For this review, take the finished solid that the model builds, in its own axes (mm). Face numbers are marked on the shaded views. A direction names the side the tool comes from. Give positions to 0.01 mm unless a question says otherwise; leave off trailing zeros. Order: outer loops, then holes, each group sorted by start corner. A loop starts at its lowest first (then second) coordinate and runs counter-clockwise, first axis right, second up. Notation, with made-up numbers: M 21.5,64.5 L 47.5,64.5 A28 ccw 47.5,82.5 Z; hole C -23.5,36.5 d4. An arc over 180 degrees is marked long. Answer as CSV lines item,"result". Start each with the question number.
1. Clearance check with flat-ended pins moving along their axes: P1, Ø1.1, axis at y = 3, z = -6.5, coming from the -X side; P2, Ø3, axis at y = 4, z = -1.5, coming from the +X side; P3, Ø4, axis at y = 2.5, z = 2, coming from the -X side. State where each tip first meets the part, or that it passes through.
2. We need section B-B, the plane z = -1. State how many separate pieces and enclosed holes the cut face has, and give its area (3 significant figures).
3. Mouldability with a two-part tool opening along Z and no side actions: class the marked faces 4, 5 and 6 as pulls with the +Z half, pulls with the -Z half, needs draft (parallel to the pull), parting line crosses it, or undercut.
4. We need section A-A, the plane x = 28. Give the boundary of the cut face in (y, z), and give its area (3 significant figures).
5. For line 1 along Z through (x, y) = (-28.5, 3.25); line 2 along X through (y, z) = (2.25, 4); line 3 along X through (y, z) = (2.75, 1.75), list the stretches that pass through material, from the lowest coordinate up.
6. Machinability: for the marked faces 1, 2 and 3, which of the approach directions +Z, -Z, +X, -X, +Y, -Y give a long, thin tool a straight path to every point of the face, cutting with its end or side? Answer none if there is none.
from build123d import *

# Parameters (mm, degrees)
SKETCH1_W           = 70
SKETCH1_H           = 16
BOSS_EXTRUDE1_DEPTH = 7
CUT_EXTRUDE1_DEPTH  = 17
SKETCH3_R           = 2
BOSS_EXTRUDE2_DEPTH = 14
SKETCH4_W           = 39
SKETCH4_H           = 10
CUT_EXTRUDE2_DEPTH  = 2
FILLET1_R           = 1
FILLET2_R           = 3.5


with BuildPart() as part:
    # Sketch1 → Boss-Extrude1 (new body)
    with BuildSketch(Plane(origin=(0, 0, 0), x_dir=(1, 0, 0), z_dir=(0, 1, 0))):
        Rectangle(SKETCH1_W, SKETCH1_H)
    extrude(amount=BOSS_EXTRUDE1_DEPTH)

    # Sketch2 → Cut-Extrude1 (cut)
    with BuildSketch(Plane(origin=(0, 7, 0), x_dir=(1, 0, 0), z_dir=(0, 1, 0))):
        Polygon((-30, 7), (-35, 7), (-35, -7), (-30, -7), (-30, -5), (-23, -5), (-23, 5), (-30, 5), align=None)
        Polygon((30, -5), (30, -7), (35, -7), (35, 7), (30, 7), (30, 5), (23, 5), (23, -5), align=None)
    extrude(amount=-CUT_EXTRUDE1_DEPTH, mode=Mode.SUBTRACT)

    # Sketch3 → Boss-Extrude2 (add)
    with BuildSketch(Plane.XY.offset(-7)):
        with Locations((-32.5, 3.5)):
            Circle(SKETCH3_R)
        with Locations(Location((32.5, 3.5, 0), (0, 0, 180))):
            Circle(SKETCH3_R)
    extrude(amount=BOSS_EXTRUDE2_DEPTH)

    # Sketch4 → Cut-Extrude2 (cut)
    with BuildSketch(Plane(origin=(0, 7, 0), x_dir=(1, 0, 0), z_dir=(0, 1, 0))):
        Rectangle(SKETCH4_W, SKETCH4_H)
    cut_extrude2 = extrude(amount=-CUT_EXTRUDE2_DEPTH, mode=Mode.SUBTRACT)

    # Mirror1: Cut-Extrude2 across plane
    add(cut_extrude2.mirror(Plane.ZX.offset(3.5)), mode=Mode.SUBTRACT)

    # Fillet1
    fillet1_edges = [part.edges().sort_by_distance(p)[0] for p in [
        (19.5, 0, 0),
        (0, 0, -5),
        (-19.5, 0, 0),
        (0, 0, 5),
        (19.5, 2, 0),
        (0, 2, -5),
        (-19.5, 2, 0),
        (0, 2, 5),
        (26.5, 0, -5),
        (23, 0, 0),
        (26.5, 0, 5),
        (-26.5, 0, -5),
        (-23, 0, 0),
        (-26.5, 0, 5),
        (-23, 7, 0),
        (-30, 3.5, 5),
        (-30, 3.5, -5),
        (-26.5, 7, -5),
        (-26.5, 7, 5),
        (26.5, 7, 5),
        (26.5, 7, -5),
        (23, 7, 0),
        (19.5, 5, 0),
        (19.5, 6, -5),
        (0, 5, 5),
        (-19.5, 5, 0),
        (0, 5, -5),
        (-19.5, 6, -5),
        (19.5, 7, 0),
        (0, 7, -5),
        (-19.5, 7, 0),
        (0, 7, 5),
    ]]
    fillet(fillet1_edges, radius=FILLET1_R - 0.0001)  # a hair under: the kernel refuses the full size

    # Fillet2
    fillet2_edges = [part.edges().sort_by_distance(p)[0] for p in [
        (-35, 7, 7.5),
        (-35, 0, 7.5),
        (-35, 0, -7.5),
        (-35, 7, -7.5),
        (35, 0, -7.5),
        (35, 7, -7.5),
        (35, 0, 7.5),
        (35, 7, 7.5),
    ]]
    fillet(fillet2_edges, radius=FILLET2_R - 0.0001)  # a hair under: the kernel refuses the full size


solid = part.part
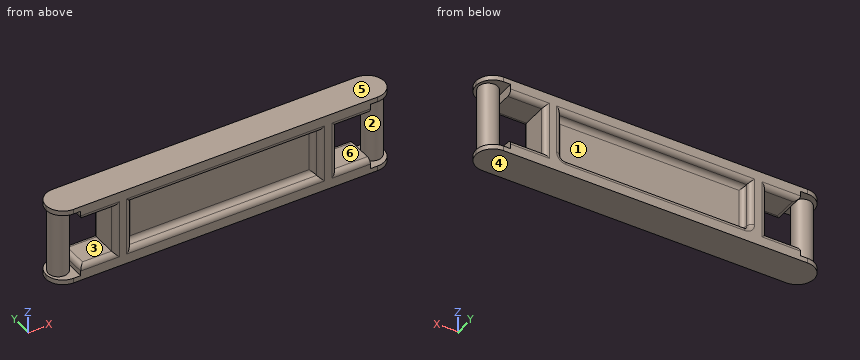
Result set:
1,P1,"x = -34.99"
1,P2,"x = 34.5"
1,P3,"x = -34.5"
2,separate pieces,"3"
2,enclosed holes,"0"
2,area,"190 mm2"
3,face 4,"pulls with the -Z half"
3,face 5,"pulls with the +Z half"
3,face 6,"undercut"
4,outline,"M 0,-8 L 7,-8 L 7,-6 A1 ccw 6,-5 L 1,-5 A1 ccw 0,-6 Z; M 0,6 A1 ccw 1,5 L 6,5 A1 ccw 7,6 L 7,8 L 0,8 Z"
4,area,"41.1 mm2"
5,line 1,"-8 to -5, 5 to 8"
5,line 2,"-34.06 to -30.94, -23 to 23, 30.94 to 34.06"
5,line 3,"-34.35 to -30.65, -23 to 23, 30.65 to 34.35"
6,face 1,"+Y"
6,face 2,"none"
6,face 3,"+Y, -Y"
